Can you work these out from the drawing? Everything is in mm from the part's minimum corner. Round coordinates to 2 decimals unless told otherwise and drop trailing zeros. Write each loop counter-clockwise with the first axis right and the second up, starting at its lowest first coordinate (ties: lowest second). Pieces come first, ordered by that corner, then holes.
Q1. Please list where these lines run through material, in increasing order: line 1 along X through (y, z) = (9, 3); line 2 along X through (y, z) = (18.75, 4.35); line 3 along Z through (x, y) = (3.25, 1.5).
Q2. If we section it at C-C (z = 4.9): Please give me the cut outline in (x, y), plus the area to 3 significant figures.
Q3. We'd pull the mould along Z, two halves only. Please class the marked faces 1, 2 and 3: +Z half, -Z half, draft (parallel to the pull), parting line (faces both ways), or undercut.
Q4. If we section it at B-B (y = 3.5): Please give me the cut outline in (x, z), plus the area to 3 significant figures.
Q5. If we section it at A-A (x = 5): Please give me the cut outline in (y, z).
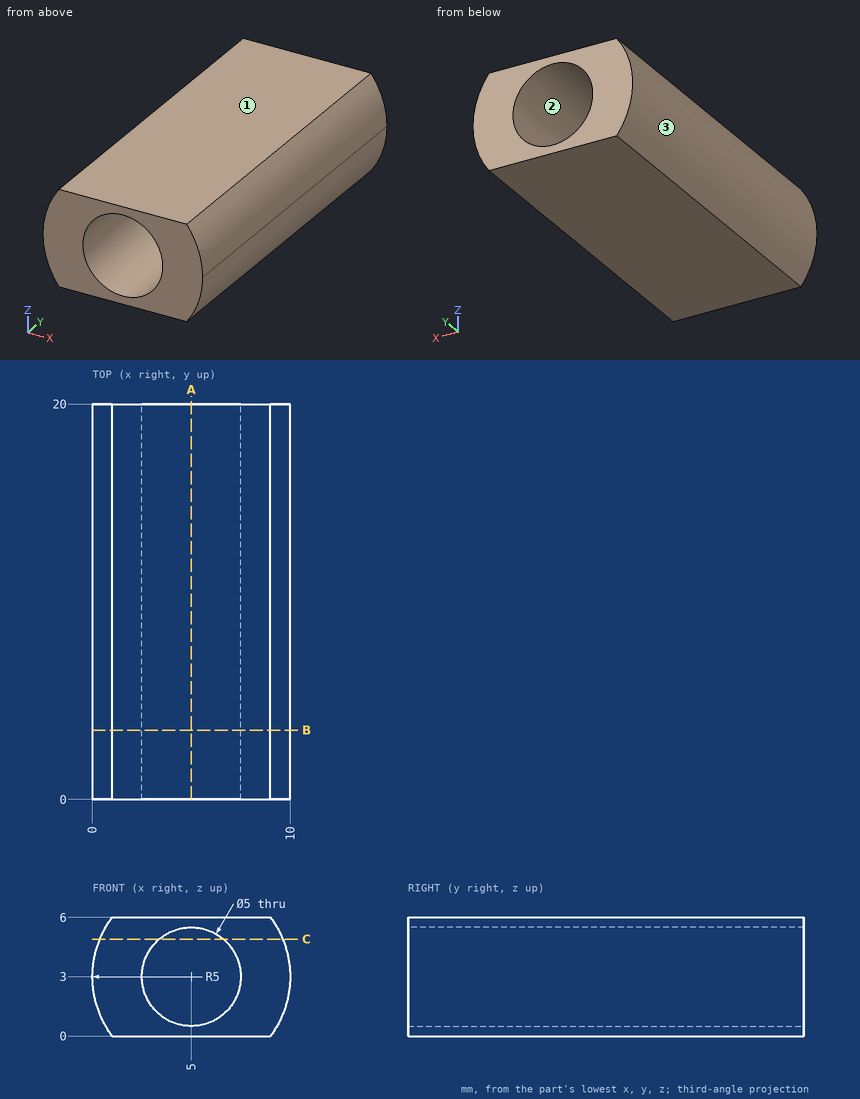
A:
1. line 1: x = 0 to 2.5, 7.5 to 10
1. line 2: x = 0.19 to 2.9, 7.1 to 9.81
1. line 3: z = 0 to 1.21, 4.79 to 6
2. outline: (0.38, 0) - (3.38, 0) - (3.38, 20) - (0.38, 20) - close; (6.62, 0) - (9.62, 0) - (9.62, 20) - (6.62, 20) - close
2. area: 120 mm2
3. face 1: +Z half
3. face 2: undercut
3. face 3: parting line
4. outline: (1, 0) - (9, 0) arc R5 ccw to (9, 6) - (1, 6) arc R5 ccw to start; hole circle Ø5 at (5, 3)
4. area: 36.5 mm2
5. outline: (0, 0) - (20, 0) - (20, 0.5) - (0, 0.5) - close; (0, 5.5) - (20, 5.5) - (20, 6) - (0, 6) - close
